```python
from build123d import *

# Parameters (mm, degrees)
SKETCH1_R           = 25
SKETCH1_R_2         = 7
SKETCH1_R_3         = 1.7
BOSS_EXTRUDE1_DEPTH = 10
SKETCH2_R           = 9.53
CUT_EXTRUDE1_DEPTH  = 8
SKETCH4_R           = 3
CUT_EXTRUDE2_DEPTH  = 7


with BuildPart() as part:
    # Sketch1 → Boss-Extrude1 (new body)
    with BuildSketch(Plane(origin=(0, 0, 0), x_dir=(1, 0, 0), z_dir=(0, 1, 0))):
        with Locations(Location((0, 0, 0), (0, 0, 270))):
            Circle(SKETCH1_R)
        with Locations(Location((0, 0, 0), (0, 0, 270))):
            Circle(SKETCH1_R_2, mode=Mode.SUBTRACT)
        with Locations(Location((0, 18, 0), (0, 0, 270))):
            Circle(SKETCH1_R_3, mode=Mode.SUBTRACT)
        with Locations(Location((18, 0, 0), (0, 0, 270))):
            Circle(SKETCH1_R_3, mode=Mode.SUBTRACT)
        with Locations(Location((0, -18, 0), (0, 0, 270))):
            Circle(SKETCH1_R_3, mode=Mode.SUBTRACT)
        with Locations(Location((-18, 0, 0), (0, 0, 270))):
            Circle(SKETCH1_R_3, mode=Mode.SUBTRACT)
    extrude(amount=BOSS_EXTRUDE1_DEPTH)

    # Sketch2 → Cut-Extrude1 (cut)
    with BuildSketch(Plane.XZ):
        with Locations(Location((0, 0, 0), (0, 0, 270))):
            Circle(SKETCH2_R)
    extrude(amount=-CUT_EXTRUDE1_DEPTH, mode=Mode.SUBTRACT)

    # Sketch4 → Cut-Extrude2 (cut)
    with BuildSketch(Plane.XZ):
        with Locations(Location((0, 18, 0), (0, 0, 270))):
            Circle(SKETCH4_R)
        with Locations(Location((-18, 0, 0), (0, 0, 270))):
            Circle(SKETCH4_R)
        with Locations(Location((0, -18, 0), (0, 0, 270))):
            Circle(SKETCH4_R)
        with Locations(Location((18, 0, 0), (0, 0, 270))):
            Circle(SKETCH4_R)
    extrude(amount=-CUT_EXTRUDE2_DEPTH, mode=Mode.SUBTRACT)


solid = part.part
```
Can you work these out from the model? Positions are in its coordinate system, mm. A direction names the side the tool comes from. Give positions to 0.01 mm unless a question says otherwise; leave off trailing zeros. Order: outer loops, then holes, each group sorted by start corner. A loop starts at its lowest first (then second) coordinate and runs counter-clockwise, first axis right, second up. Notation, with made-up numbers: (58, -34.5) - (77, -34.5) arc R19 ccw to (77, -25.5) - close; hole circle Ø4 at (73.25, 47.5). An arc over 180 degrees is marked (long way). Use a Markdown table: item, result. Add a question column.
Q1. On a 3-axis mill with a long thin cutter (end or side, diameter ignored), from which of +Z, -Z, +X, -X, +Y, -Y can I reach the whole of each face in a straight line? I mean faces 1 (the cylindrical face through (-5.8, 3.94, 7.56)), 2 (the cylindrical face through (-0.65, 8.48, -16.43)). Say none if no direction works.
Q2. If we section it at A-A on x = 0: Write out the boundary of the cut face in (y, z).
Q3. If we section it at C-C on z = 18: Write out the boundary of the cut face in (x, y).
Q4. Please list where these lines run through material, in increasing order: line 1 along X through (y, z) = (9.35, 0); line 2 along X through (y, z) = (4.5, 0); line 3 along X through (y, z) = (9.75, -2.5).
Q5. If we section it at B-B on z = 0: Write out the boundary of the cut face in (x, y), plus the area to 3 significant figures.
Q6. I'm going to push flat-ended pins straight in: pin 1 (3.5 mm diameter, centred on x = 18, z = 0, fed in from -Y); pin 2 (3 mm diameter, centred on x = 5.5, y = 8, fed in from -Z); pin 3 (1 mm diameter, centred on x = -14, y = 5, fed in from -Z); pin 4 (3 mm diameter, centred on x = 0, z = 18, fed in from -Y). Where does each tip first touch, or does it pass through?
Q7. If we section it at D-D on x = 5.5: Write out the boundary of the cut face in (y, z).
Q8. If we mould it in two halves opening along Z, with no side actions, what happens to faces 3 (the flat face through (-11, 0, 0)), 4 (the cylindrical face through (0, 3, -15)), 5 (the cylindrical face through (7.509, 4.93, 23.846))? For each: released by +Z, released by -Z, zero draft, split by the parting line, or undercut.
Answers follow:
| question | item | result |
|---|---|---|
| 1 | face 1 | -Y |
| 1 | face 2 | +Y, -Y |
| 2 | outline | (0, -25) - (10, -25) - (10, -19.7) - (7, -19.7) - (7, -21) - (0, -21) - close; (0, -15) - (7, -15) - (7, -16.3) - (10, -16.3) - (10, -7) - (8, -7) - (8, -9.53) - (0, -9.53) - close; (0, 9.53) - (8, 9.53) - (8, 7) - (10, 7) - (10, 16.3) - (7, 16.3) - (7, 15) - (0, 15) - close; (0, 21) - (7, 21) - (7, 19.7) - (10, 19.7) - (10, 25) - (0, 25) - close |
| 3 | outline | (-17.35, 0) - (-3, 0) - (-3, 7) - (-1.7, 7) - (-1.7, 10) - (-17.35, 10) - close; (1.7, 7) - (3, 7) - (3, 0) - (17.35, 0) - (17.35, 10) - (1.7, 10) - close |
| 4 | line 1 | x = -25 to -19.7, -16.3 to -7, 7 to 16.3, 19.7 to 25 |
| 4 | line 2 | x = -25 to -21, -15 to -9.53, 9.53 to 15, 21 to 25 |
| 4 | line 3 | x = -24.87 to -6.54, 6.54 to 24.87 |
| 5 | outline | (-25, 0) - (-21, 0) - (-21, 7) - (-19.7, 7) - (-19.7, 10) - (-25, 10) - close; (-16.3, 7) - (-15, 7) - (-15, 0) - (-9.53, 0) - (-9.53, 8) - (-7, 8) - (-7, 10) - (-16.3, 10) - close; (7, 8) - (9.53, 8) - (9.53, 0) - (15, 0) - (15, 7) - (16.3, 7) - (16.3, 10) - (7, 10) - close; (19.7, 7) - (21, 7) - (21, 0) - (25, 0) - (25, 10) - (19.7, 10) - close |
| 5 | area | 215 mm^2 |
| 6 | pin 1 | stops at y = 7 |
| 6 | pin 2 | stops at z = -24.68 |
| 6 | pin 3 | stops at z = -21.04 |
| 6 | pin 4 | passes through |
| 7 | outline | (0, -24.39) - (10, -24.39) - (10, -4.33) - (8, -4.33) - (8, -7.78) - (0, -7.78) - close; (0, 7.78) - (8, 7.78) - (8, 4.33) - (10, 4.33) - (10, 24.39) - (0, 24.39) - close |
| 8 | face 3 | zero draft |
| 8 | face 4 | undercut |
| 8 | face 5 | split by the parting line |
